```python
from build123d import *

# Parameters (mm, degrees)
F0_R     = 40
F1_DEPTH = 5
F3_D     = 5.5
F4_SIZE  = 1


with BuildPart() as f1:
    # F0 (on Top) → F1 (new body)
    with BuildSketch(Plane.XY):
        Circle(F0_R)
    extrude(amount=F1_DEPTH)

    # F3 (through all)
    with Locations(Plane(origin=(0, 0, 0), x_dir=(1, 0, 0), z_dir=(0, 0, -1))):
        with Locations((0, 30), (25.980762, -15), (-25.980762, -15)):
            Hole(F3_D / 2)

    # F4
    f4_edges = [f1.edges().sort_by_distance(p)[0] for p in [
        (-40, 0, 5),
        (-40, 0, 0),
    ]]
    chamfer(f4_edges, length=F4_SIZE)


solid = f1.part
```
Check sheet for the modelled part. Datum: model origin and axes. Units: mm. Give positions to 0.01 mm unless a question says otherwise; leave off trailing zeros. Loops run counter-clockwise (first coordinate to the right, second up) from the corner with the lowest first, then second, coordinate; pieces in that order, holes last. Notation, with made-up numbers: M 33.5,83.25 L 88.5,83.25 A20 cw 88.5,102.25 Z; hole C -30.75,6.5 d11. An arc over 180 degrees is marked long. Answer in a Markdown table with one row per item.
1) Thickness scan on line 1 (X direction, y = 15, z = 1.9); line 2 (Y direction, x = 0, z = 3.1); line 3 (X direction, y = -30, z = 1.55). Record the ranges inside material, lowest first.
Solutions:
| item | result |
|---|---|
| line 1 | x = -37.08 to -28.73, -23.23 to 23.23, 28.73 to 37.08 |
| line 2 | y = -40 to -32.75, -27.25 to 40 |
| line 3 | x = -26.46 to -2.75, 2.75 to 26.46 |
2) Cross-section at B-B (y = 15). Count the separate pieces of the cut face and the enclosed holes in it, plus the area to 3 significant figures.
Solutions:
| item | result |
|---|---|
| separate pieces | 3 |
| enclosed holes | 0 |
| area | 314 mm^2 |
3) Mould release check, pull along Y, two halves, no side actions. Record for faces 1 (the face through (-1, 1, 5)), 2 (the face through (-8.67, -39.05, 2.48)), 3 (the face through (-28.604, 14.174, 2.535)): released by +Y, released by -Y, zero draft, split by the parting line, or undercut.
Solutions:
| item | result |
|---|---|
| face 1 | zero draft |
| face 2 | split by the parting line |
| face 3 | undercut |
4) Depth check by flat-ended pin: pin 1 (1.5 mm diameter, centred on x = 2.5, z = 3, fed in from +Y); pin 2 (5 mm diameter, centred on x = -25.98, y = 15, fed in from -Z); pin 3 (1 mm diameter, centred on x = -29, z = 1.5, fed in from +Y); pin 4 (2 mm diameter, centred on x = 24.5, y = 32, fed in from +Z). Enter the tip coordinate at first touch or a pass-through.
Solutions:
| item | result |
|---|---|
| pin 1 | stops at y = 39.96 |
| pin 2 | passes through |
| pin 3 | stops at y = 28.07 |
| pin 4 | stops at z = 4.7 |
5) Cross-section at A-A (x = 0). Enter the section's corners in (y, z).
Solutions:
| item | result |
|---|---|
| outline | M -40,1 L -39,0 L -32.75,0 L -32.75,5 L -39,5 L -40,4 Z; M -27.25,0 L 39,0 L 40,1 L 40,4 L 39,5 L -27.25,5 Z |
